The listing builds one solid part. Answer for the finished solid, in the listing's coordinates (mm). Face numbers are marked on the shaded views. A direction names the side the tool comes from. Coordinates: 2 decimals unless noted, no trailing zeros. Loops run counter-clockwise (first coordinate to the right, second up) from the corner with the lowest first, then second, coordinate; pieces in that order, holes last. Notation, with made-up numbers: (-27, 57.5) - (-4, 57.5) arc R13 ccw to (-4, 75.5) - close; hole circle Ø10 at (-37, -17.5). An arc over 180 degrees is marked (long way). Return JSON: item names as keys, results as strings. Group by question number.
1. The mould has two halves that part along Z. Classify the marked faces 5, 6, 7 and 8: pulls with the +Z half, pulls with the -Z half, needs draft (parallel to the pull), parting line crosses it, or undercut.
2. Section B-B (y = -5.75) is taken. Write down the section's boundary in (x, z).
3. Each of these flat-tipped pins is pushed along its axis until it touches: P1, Ø4, axis at x = 6.5, y = 4, coming from the -Z side; P2, Ø3, axis at x = 5, z = -0.5, coming from the -Y side; P3, Ø1.5, axis at x = 2.5, z = -1.5, coming from the +Y side. Where does it stop, or does it pass through?
4. Which of the six approach directions +Z, -Z, +X, -X, +Y, -Y give full straight-line access (tool end or side, diameter ignored) to the marked faces 1, 2, 3 and 4?
5. Find the intervals of material crossed by line 1 along Y through (x, z) = (2, 0); line 2 along Y through (x, z) = (5, 0); line 3 along X through (y, z) = (1.5, -5), in increasing order.
6. Section A-A (x = 6.75) is taken. Write down the section's boundary in (y, z), and give its area (3 significant figures).
7. Section C-C (z = -6) is taken. Write down the section's boundary in (x, y), and give its area (3 significant figures).
```python
from build123d import *

# Parameters (mm, degrees)
SKETCH1_R      = 2.5
EXTRUDE1_DEPTH = 9
SKETCH3_W      = 3
SKETCH3_H      = 4.5


# Read off the part's stored shape, not the designer's step: Cut-Extrude1
with BuildPart() as part:
    # Sketch1 → Extrude1 (new body)
    with BuildSketch(Plane(origin=(0, 0, 0), x_dir=(0, 0, -1), z_dir=(1, 0, 0))):
        Polygon((5.773502692, 0), (2.886751346, 5), (-2.886751346, 5), (-5.773502692, 0), (-2.886751346, -5), (2.886751346, -5), align=None)
        Circle(SKETCH1_R, mode=Mode.SUBTRACT)
    extrude(amount=EXTRUDE1_DEPTH)

    # Cut-Extrude1 outline → Cut-Extrude1 (revolve, cut)
    with BuildSketch(Plane.YX):
        Polygon((5.773502692, 9.000000845), (4.99999886, 9.000000845), (5.773502688, 8.553418015), align=None)
    revolve(axis=Axis((0, 0, 0), (1, 0, 0)), mode=Mode.SUBTRACT)

    # Sketch3 → Revolve1 (revolve)
    with BuildSketch(Plane.XY, mode=Mode.PRIVATE) as revolve1_sk:
        with Locations((1.5, 4.75)):
            Rectangle(SKETCH3_W, SKETCH3_H)
    revolve(revolve1_sk.sketch.rotate(Axis((0, 0, 0), (-1, 0, 0)), 90), axis=Axis((0, 0, 0), (-1, 0, 0)))


solid = part.part
```
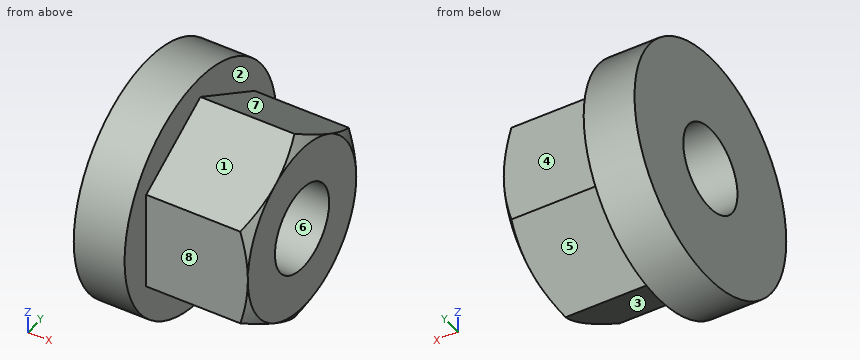
The answers:
{
 "1": {"face 5": "pulls with the -Z half", "face 6": "undercut", "face 7": "pulls with the +Z half", "face 8": "needs draft"},
 "2": {"outline": "(0, -3.99) - (3, -3.99) - (3, 3.99) - (0, 3.99) - close"},
 "3": {"P1": "stops at z = -4.62", "P2": "stops at y = -5", "P3": "stops at y = 6.96"},
 "4": {"face 1": "+Z, +X, -Y", "face 2": "+X", "face 3": "-Z, +X, -Y", "face 4": "+Z, -Z, +X, +Y"},
 "5": {"line 1": "y = -7 to -2.5, 2.5 to 7", "line 2": "y = -5 to -2.5, 2.5 to 5", "line 3": "x = 0 to 3"},
 "6": {"outline": "(-5, -2.89) - (0, -5.77) - (5, -2.89) - (5, 2.89) - (0, 5.77) - (-5, 2.89) - close; hole circle Ø5 at (0, 0)", "area": "67.0 mm2"},
 "7": {"outline": "(0, -3.61) - (3, -3.61) - (3, 3.61) - (0, 3.61) - close", "area": "21.6 mm2"}
}
